Design review of the part built by this model. Coordinates are the model's own, in mm. Coordinates: 2 decimals unless noted, no trailing zeros. Loops run counter-clockwise (first coordinate to the right, second up) from the corner with the lowest first, then second, coordinate; pieces in that order, holes last. Notation, with made-up numbers: (-13.5, 19) - (40.5, 19) arc R26 cw to (40.5, 34) - close; hole circle Ø1 at (19, 21.5). An arc over 180 degrees is marked (long way). Use one line per item in the form item = value. Start each with the question number.
(1) Clearance check with flat-ended pins moving along their axes: pin 1 Ø3 at (x, y) = (193.5, 4) entering from -Z; pin 2 Ø1 at (x, z) = (79, -43) entering from -Y; pin 3 Ø1.9 at (y, z) = (3, 244) entering from +X; pin 4 Ø1.9 at (y, z) = (2, 245.5) entering from -X. State where each tip first meets the part, or that it passes through.
(2) Add section A-A (z = 118). State the section outline as (x, y) points.
(3) For L1, parallel to X at y = 4.5, z = 132.5, list the stretches that pass through material, from the lowest coordinate up.
(4) Add section B-B (x = 100). State the section outline as (y, z) points.
(5) Add section C-C (y = 4). Count the separate pieces of the cut face and the enclosed holes in it, plus the area to 3 significant figures.
```python
from build123d import *

# Parameters (mm, degrees)
SKETCH2_W           = 400
SKETCH2_H           = 500
BOSS_EXTRUDE2_DEPTH = 6.35
CHAMFER1_SIZE       = 25
SKETCH9_W           = 6.35
SKETCH9_H           = 36
SKETCH9_W_2         = 36
SKETCH9_H_2         = 6.35
CUT_EXTRUDE1_DEPTH  = 321.219178845


with BuildPart() as part:
    # Sketch2 → Boss-Extrude2 (new body)
    with BuildSketch(Plane(origin=(0, 0, 0), x_dir=(1, 0, 0), z_dir=(0, 1, 0))):
        Rectangle(SKETCH2_W, SKETCH2_H)
    extrude(amount=BOSS_EXTRUDE2_DEPTH)

    # Chamfer1
    chamfer1_edges = [part.edges().sort_by_distance(p)[0] for p in [
        (200, 3.175, 250),
        (-200, 3.175, 250),
        (-200, 3.175, -250),
        (200, 3.175, -250),
    ]]
    chamfer(chamfer1_edges, length=CHAMFER1_SIZE)

    # Sketch9 → Cut-Extrude1 (cut, through all)
    with BuildSketch(Plane(origin=(0, 6.35, 0), x_dir=(1, 0, 0), z_dir=(0, 1, 0))):
        with Locations((194.825, 117)):
            Rectangle(SKETCH9_W, SKETCH9_H)
        with Locations((102, -244.825)):
            Rectangle(SKETCH9_W_2, SKETCH9_H_2)
        with Locations((-102, -244.825)):
            Rectangle(SKETCH9_W_2, SKETCH9_H_2)
        with Locations((-102, 244.825)):
            Rectangle(SKETCH9_W_2, SKETCH9_H_2)
        with Locations((102, 244.825)):
            Rectangle(SKETCH9_W_2, SKETCH9_H_2)
        with Locations((194.825, -117)):
            Rectangle(SKETCH9_W, SKETCH9_H)
        with Locations((-194.825, -117)):
            Rectangle(SKETCH9_W, SKETCH9_H)
        with Locations((-194.825, 117)):
            Rectangle(SKETCH9_W, SKETCH9_H)
    extrude(amount=-CUT_EXTRUDE1_DEPTH, mode=Mode.SUBTRACT)


solid = part.part
```
Computed values:
q1.pin_1 = -233
q1.pin_2 = 0
q1.pin_3 = 181.95
q1.pin_4 = -180.45
q2.outline = (-200, 0) - (-198, 0) - (-198, 6.35) - (-200, 6.35) - close; (-191.65, 0) - (191.65, 0) - (191.65, 6.35) - (-191.65, 6.35) - close; (198, 0) - (200, 0) - (200, 6.35) - (198, 6.35) - close
q3.L1 = -200 to -198, -191.65 to 191.65, 198 to 200
q4.outline = (0, -250) - (6.35, -250) - (6.35, -248) - (0, -248) - close; (0, -241.65) - (6.35, -241.65) - (6.35, 241.65) - (0, 241.65) - close; (0, 248) - (6.35, 248) - (6.35, 250) - (0, 250) - close
q5.separate_pieces = 1
q5.enclosed_holes = 8
q5.area = 197,000 mm^2
